from build123d import *

# Parameters (mm, degrees)
F1_ANGLE_BACK  = 90
F1_ANGLE       = 180
F2_DEPTH       = 38.1
F4_DEPTH       = 19.051
F6_ANGLE_BACK  = 90
F6_ANGLE       = 180
F10_R          = 5.08
F10_R_2        = 4.445
F11_DEPTH      = 6.35
F12_DEPTH      = 2.794
F12_DEPTH_BACK = 6.35
F13_R          = 2.54


with BuildPart() as f1:
    # F0 (on Right) → F1 (revolve)
    with BuildSketch(Plane.YZ, mode=Mode.PRIVATE) as f1_sk:
        with BuildLine():
            Line((-19.05, 0), (0, 0))
            Line((0, 0), (0, 12.7))
            Line((0, 12.7), (0, 19.05))
            ThreePointArc((0, 19.05), (-9.950869572, 17.152608716), (-19.05, 12.7))
            Line((-19.05, 12.7), (-19.05, 0))
        make_face()
    revolve(f1_sk.sketch.rotate(Axis((0, 0, 6.35), (0, 0, -1)), -F1_ANGLE_BACK), axis=Axis((0, 0, 6.35), (0, 0, -1)), revolution_arc=F1_ANGLE)

    # F2 (add): a face of the model
    f2_faces = [f1.faces().sort_by_distance(p)[0] for p in [
        (0, 0, 8.5143309126),
    ]]
    extrude(f2_faces, amount=F2_DEPTH)

    # F3 (on face) → F4 (cut, through all)
    with BuildSketch(Plane(origin=(0, 0, 0), x_dir=(1, 0, 0), z_dir=(0, 0, -1))):
        with BuildLine():
            ThreePointArc((19.05, 0), (17.2317314868, -19.1462308649), (13.97, -38.1))
            Line((13.97, -38.1), (19.05, -38.1))
            Line((19.05, -38.1), (19.05, 0))
        make_face()
        with BuildLine():
            Line((-19.05, -38.1), (-13.97, -38.1))
            ThreePointArc((-13.97, -38.1), (-17.2317314868, -19.1462308649), (-19.05, 0))
            Line((-19.05, 0), (-19.05, -38.1))
        make_face()
    extrude(amount=-F4_DEPTH, mode=Mode.SUBTRACT)

    # F5 (on Right) → F6 (revolve, cut)
    with BuildSketch(Plane.YZ, mode=Mode.PRIVATE) as f6_sk:
        Polygon((32.9955678842, 19.05), (38.1, 0), (45.72, 0), (45.72, 19.05), (38.1, 19.05), align=None)
    revolve(f6_sk.sketch.rotate(Axis((0, -19.05, 6.35), (0, 0, -1)), -F6_ANGLE_BACK), axis=Axis((0, -19.05, 6.35), (0, 0, -1)), revolution_arc=F6_ANGLE, mode=Mode.SUBTRACT)

    # F7 (on Right) → F8 (revolve, cut)
    with BuildSketch(Plane.YZ):
        with BuildLine():
            ThreePointArc((-4.4901280605, 14.5598719395), (0, 12.7), (4.4901280605, 14.5598719395))
            Line((4.4901280605, 14.5598719395), (19.18810552, 29.2578493989))
            Line((19.18810552, 29.2578493989), (14.6979774594, 33.7479774594))
            Line((14.6979774594, 33.7479774594), (-4.4901280605, 14.5598719395))
        make_face()
    revolve(axis=Axis((0, 17.5408982918, 36.5908982918), (0, 0.7071067812, 0.7071067812)), mode=Mode.SUBTRACT)

    # F10 (on offset) → F11 (cut)
    with BuildSketch(Plane.XY.offset(15.2654)):
        Circle(F10_R)
        Circle(F10_R_2, mode=Mode.SUBTRACT)
        Circle(F10_R_2)
    extrude(amount=-F11_DEPTH, mode=Mode.SUBTRACT)

    # F10 (on offset) → F12 (join, two sides)
    with BuildSketch(Plane.XY.offset(15.2654)) as f12_sk:
        Circle(F10_R_2)
    extrude(amount=F12_DEPTH)
    extrude(f12_sk.sketch, amount=-F12_DEPTH_BACK)

    # F13
    f13_edges = [f1.edges().sort_by_distance(p)[0] for p in [
        (-4.445, 0, 18.0594),
    ]]
    fillet(f13_edges, radius=F13_R)


solid = f1.part
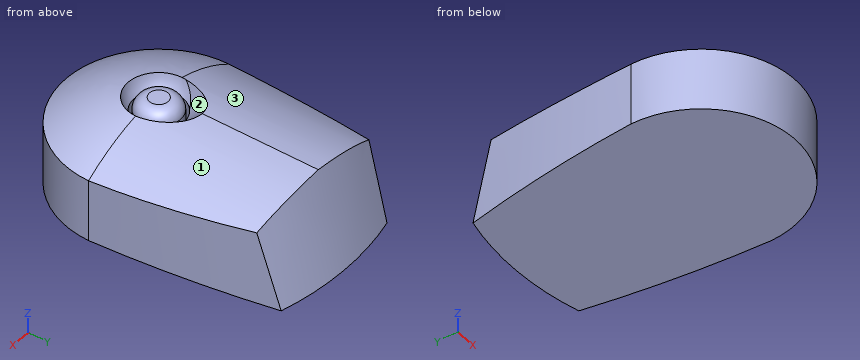
Design review of the part built by this model. Coordinates are the model's own, in mm. Face numbers are marked on the shaded views. Coordinates: 2 decimals unless noted, no trailing zeros. Loops run counter-clockwise (first coordinate to the right, second up) from the corner with the lowest first, then second, coordinate; pieces in that order, holes last. Notation, with made-up numbers: M 32,27.25 L 41,27.25 A19 ccw 41,39.25 Z; hole C 25,66.25 d9. An arc over 180 degrees is marked long. Use one line per item in the form item = value.
(1) Clearance check with flat-ended pins moving along their axes: P1, Ø8, axis at x = 0, y = -2, coming from the +Z side; P2, Ø5, axis at x = -8.5, z = 10.5, coming from the +Y side; P3, Ø1, axis at x = 9.5, z = 16.5, coming from the +Y side. State where each tip first meets the part, or that it passes through.
Return value:
P1 = 18.06
P2 = 35.39
P3 = 32.98
(2) Consider section A-A (y = 13). Write out the cut boundary in (x, z).
Return value:
outline = M -17.98,0 L 17.98,0 L 17.98,13.39 A38.1 ccw 0,19.05 A38.1 ccw -17.98,13.39 Z
(3) For line 1 along Y through (x, z) = (0, 13) (3 decimals); line 2 along Y through (x, z) = (0, 12.75) (3 decimals); line 3 along X through (y, z) = (-7.5, 7), list the stretches that pass through material, from the lowest coordinate up. Write a range as from..to.
Return value:
line_1 = -18.593..-5.08, -4.445..4.445, 5.08..34.617
line_2 = -18.975..-5.08, -4.445..4.445, 5.08..34.684
line_3 = -17.51..17.51
(4) Consider section B-B (z = 6.5). Write out the cut boundary in (x, y).
Return value:
outline = M -19.05,0 A19.05 ccw 19.05,0 A254 ccw 14.73,34.36 A55.41 ccw -14.73,34.36 A254 ccw Z
(5) Draft analysis for pull direction X (two halves, no side actions). For the marked faces 1, 2 and 3, state which applies: pulls with the +X half, pulls with the -X half, needs draft (parallel to the pull), parting line crosses it, or undercut.
Return value:
face_1 = pulls with the +X half
face_2 = undercut
face_3 = pulls with the -X half
